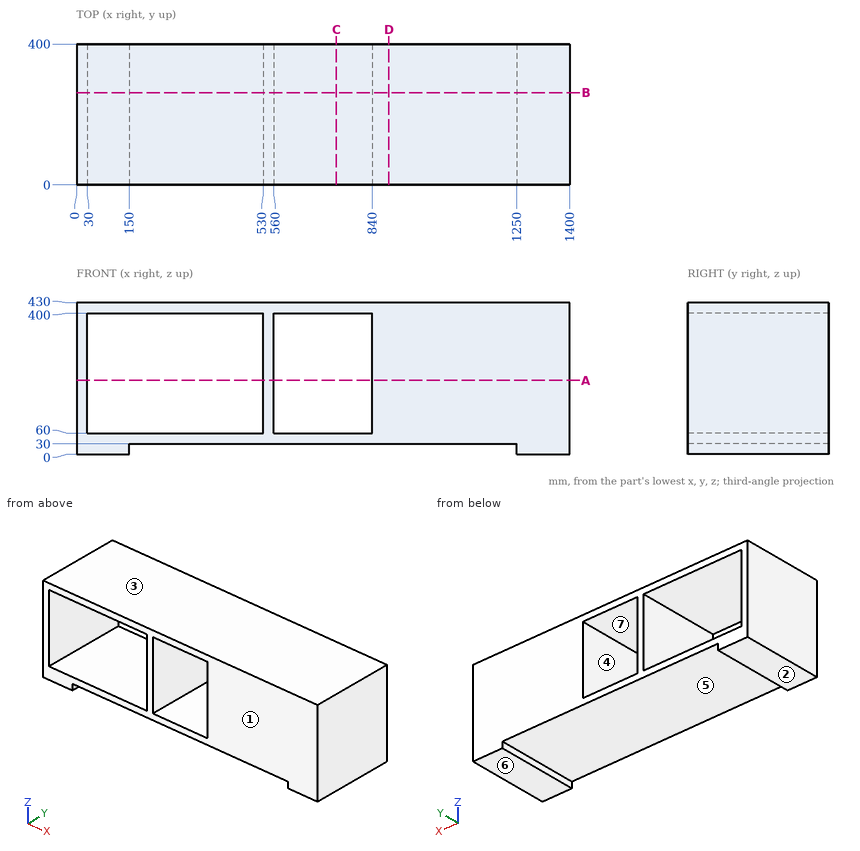
Can you work these out from the drawing? Everything is in mm from the part's minimum corner. A direction names the side the tool comes from. Round coordinates to 2 decimals unless told otherwise and drop trailing zeros. Loops run counter-clockwise (first coordinate to the right, second up) from the corner with the lowest first, then second, coordinate; pieces in that order, holes last. Notation, with made-up numbers: M 56,23.5 L 112,23.5 A14 cw 112,49.5 Z; hole C 50.5,48 d1. An arc over 180 degrees is marked long. Write item = value, one per line.
1. I want a section at B-B, the plane y = 262. Write out the boundary of the cut face in (x, z), and give its area (3 significant figures).
Results below:
outline = M 0,0 L 150,0 L 150,30 L 1250,30 L 1250,0 L 1400,0 L 1400,430 L 0,430 Z; hole M 30,60 L 530,60 L 530,400 L 30,400 Z; hole M 560,60 L 840,60 L 840,400 L 560,400 Z
area = 304,000 mm²
2. I want a section at A-A, the plane z = 210. Write out the boundary of the cut face in (x, y), and give its area (3 significant figures).
Results below:
outline = M 0,0 L 30,0 L 30,400 L 0,400 Z; M 530,0 L 560,0 L 560,400 L 530,400 Z; M 840,0 L 1400,0 L 1400,400 L 840,400 Z
area = 248,000 mm²
3. I want a section at D-D, the plane x = 887. Write out the boundary of the cut face in (y, z).
Results below:
outline = M 0,30 L 400,30 L 400,430 L 0,430 Z
4. I need wall thicknesses on probe 1 along X at (y, z) = (163.5, 179); probe 2 along Z at (x, y) = (503.5, 263); probe 3 along Z at (x, y) = (136, 127). Which ranges of each line are inside material? Lowest first, please.
Results below:
probe_1 = 0 to 30, 530 to 560, 840 to 1400
probe_2 = 30 to 60, 400 to 430
probe_3 = 0 to 60, 400 to 430
5. Which directions (+Z, -Z, +X, -X, +Y, -Y) give clear straight access to the entire face, cutting with the end or side of a thin tool? Please do the marked faces 5, 6 and 7.
Results below:
face_5 = -Z, +Y, -Y
face_6 = -Z, +X, -X, +Y, -Y
face_7 = +Y, -Y
6. I want a section at C-C, the plane x = 737.5. Write out the boundary of the cut face in (y, z).
Results below:
outline = M 0,30 L 400,30 L 400,60 L 0,60 Z; M 0,400 L 400,400 L 400,430 L 0,430 Z
7. Will these pins go through, and if not, where does the flat tip stop? P1, Ø9, axis at y = 280.5, z = 16.5, coming from the -X side; P2, Ø10, axis at x = 225.5, y = 76.5, coming from the -Z side.
Results below:
P1 = 0
P2 = 30
8. Thinking about a two-plate mould opening in Z: for the marked faces 1, 2, 3 and 4, which applies, +Z half, -Z half, draft (parallel to the pull), parting line (faces both ways), or undercut?
Results below:
face_1 = draft
face_2 = -Z half
face_3 = +Z half
face_4 = undercut
